Can you work these out from the model? Positions are in its coordinate system, mm. A direction names the side the tool comes from. Round coordinates to 2 decimals unless told otherwise and drop trailing zeros. Loops run counter-clockwise (first coordinate to the right, second up) from the corner with the lowest first, then second, coordinate; pieces in that order, holes last.
(1) Thinking about a two-plate mould opening in X: for faces 5 (the face through (0.142, 5.567, -6.476)), 6 (the face through (0.05, 19.51, -2.34)), 7 (the face through (5, 11, 0)), 8 (the face through (3.7, 14.59, -3.07)), which applies, released by +X, released by -X, zero draft, split by the parting line, or undercut?
(2) Will these pins go through, and if not, where does the flat tip stop? pin 1 Ø6 at (x, y) = (3.5, 17) entering from -Z; pin 2 Ø4 at (x, y) = (-3.5, 13) entering from +Z; pin 3 Ø5 at (x, y) = (1, 9) entering from -Z.
(3) If I drill on line 1 along X through (y, z) = (1.15, 0); line 2 along Y through (x, z) = (-1.5, 6); line 3 along Z through (x, y) = (1.25, 11.25), over which ranges is the centre line in solid material (lowest first)?
(4) I want a section at A-A on z = 3.5. Write out the boundary of the cut face in (x, y), plus the area to 3 significant figures.
(5) Which directions (+Z, -Z, +X, -X, +Y, -Y) give clear straight access to the entire face, cutting with the end or side of a thin tool? Please do faces 1 (the face through (4.363, 0.74, 0.573)), 2 (the face through (-5, 11, 0)), 3 (the face through (0.1, 9.9, -4.1)), 4 (the face through (1, 13.8, -4.6)).
(6) I want a section at B-B on z = 1.75. Write out the boundary of the cut face in (x, y), plus the area to 3 significant figures.
from build123d import *

# Parameters (mm, degrees)
REVOLUCI_N1_ANGLE          = 180
CROQUIS2_R                 = 7
SALIENTE_EXTRUIR1_DEPTH    = 1.5
CROQUIS3_R                 = 4.4
CORTAR_EXTRUIR1_DEPTH      = 3
CORTAR_EXTRUIR6_DEPTH      = 1
CORTAR_EXTRUIR6_DEPTH_BACK = 1


with BuildPart() as part:
    # Croquis1 → Revoluci_n1 (revolve)
    with BuildSketch(Plane.XY):
        with BuildLine():
            Line((0, 0), (0, 1.5))
            Line((0, 1.5), (5.5, 1.5))
            add(Edge.make_bspline(
                [(4.1, 9.5), (5.288924253, 7.200139579), (5.394574911, 4.30480441), (5.5, 1.5)],
                knots=[0, 0, 0, 0, 0.667768354, 0.667768354, 0.667768354, 0.667768354], degree=3))
            Line((4.1, 9.5), (4.1, 10.258992023))
            add(Edge.make_bspline(
                [(2.1, 19.5), (3.785937607, 15.030292429), (4.1, 10.258992023)],
                knots=[0, 0, 0, 1, 1, 1], degree=2))
            Line((2.1, 19.5), (3.498445406, 19.565957924))
            Line((3.498445406, 19.565957924), (6.084400468, 9.749308612))
            Line((6.084400468, 9.749308612), (7, 0))
            Line((7, 0), (0, 0))
        make_face()
    revolve(axis=Axis((0, 1.5, 0), (0, 1, 0)), revolution_arc=REVOLUCI_N1_ANGLE)

    # Croquis2 → Saliente-Extruir1 (add)
    with BuildSketch(Plane.XZ):
        with Locations(Location((0, 0, 0), (0, 0, 270))):
            Circle(CROQUIS2_R)
    extrude(amount=-SALIENTE_EXTRUIR1_DEPTH)

    # Croquis3 → Cortar-Extruir1 (cut)
    with BuildSketch(Plane.XZ):
        with Locations(Location((0, 0, 0), (0, 0, 270))):
            Circle(CROQUIS3_R)
    extrude(amount=-CORTAR_EXTRUIR1_DEPTH, mode=Mode.SUBTRACT)

    # Croquis4 → Cortar-Extruir6 (cut, two sides: drawn at the far end of the back side and taken through both)
    with BuildSketch(Plane(origin=(0, 0, 0), x_dir=(0, 0, -1), z_dir=(1, 0, 0)).offset(-CORTAR_EXTRUIR6_DEPTH_BACK)):
        Polygon((6.768665295, 7.140982448), (6.068665295, 7.140982448), (2.336951323, 20.779679502), (3.498445406, 19.565957924), (4.898652058, 19.565957924), (8.788984747, 7.140982448), align=None)
    extrude(amount=CORTAR_EXTRUIR6_DEPTH + CORTAR_EXTRUIR6_DEPTH_BACK, mode=Mode.SUBTRACT)


solid = part.part
Filled sheet:
1. face 5: split by the parting line
1. face 6: undercut
1. face 7: zero draft
1. face 8: released by +X
2. pin 1: stops at z = -4.53
2. pin 2: stops at z = 0
2. pin 3: stops at z = -6.37
3. line 1: x = -7 to -4.4, 4.4 to 7
3. line 2: y = 0 to 1.5
3. line 3: z = -5.55 to -3.82
4. outline: (-6.06, 0) - (-2.67, 0) - (-2.67, 1.5) - (-6.06, 1.5) - close; (2.67, 0) - (6.06, 0) - (6.06, 1.5) - (2.67, 1.5) - close
4. area: 10.2 mm2
5. face 1: -Y
5. face 2: +Z, +X, -X, +Y
5. face 3: +Z, -Y
5. face 4: -Z, +Y
6. outline: (-6.78, 0) - (-4.04, 0) - (-4.04, 1.5) - (-6.78, 1.5) - close; (4.04, 0) - (6.78, 0) - (6.78, 1.5) - (4.04, 1.5) - close
6. area: 8.22 mm2
